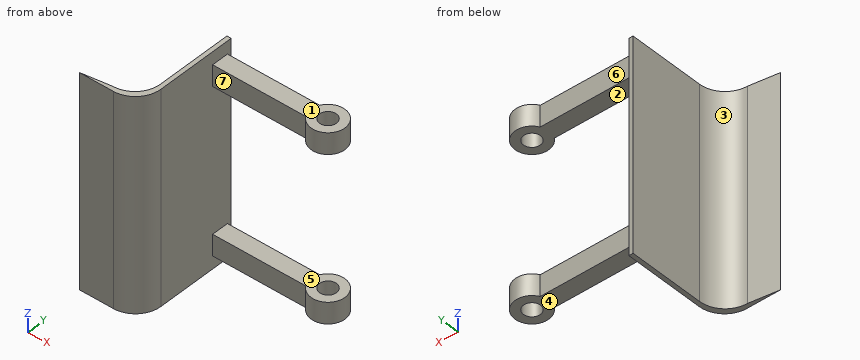
from build123d import *

# Parameters (mm, degrees)
BOSS_EXTRU_1_DEPTH      = 250
ESQUISSE3_W             = 25
ESQUISSE3_H             = 20
BOSS_EXTRU_2_DEPTH      = 125
ESQUISSE4_R             = 20
BOSS_EXTRU_3_DEPTH      = 25
ESQUISSE5_R             = 20
BOSS_EXTRU_4_DEPTH      = 25
ESQUISSE6_R             = 10
ENL_V_MAT_EXTRU_1_DEPTH = 236


with BuildPart() as part:
    # Esquisse1 → Boss.-Extru.1 (new body)
    with BuildSketch(Plane.XY):
        with BuildLine():
            Line((-30, 0), (-69.925793841, 0))
            Line((-69.925793841, 0), (-35, 5))
            ThreePointArc((-35, 5), (-13.786796564, 13.786796564), (-5, 35))
            Line((-5, 35), (-5, 125))
            Line((-5, 125), (0, 125))
            Line((0, 125), (0, 30))
            ThreePointArc((0, 30), (-8.786796564, 8.786796564), (-30, 0))
        make_face()
    extrude(amount=BOSS_EXTRU_1_DEPTH)

    # Esquisse3 → Boss.-Extru.2 (add)
    with BuildSketch(Plane(origin=(0, 0, 0), x_dir=(0, 0, -1), z_dir=(1, 0, 0))):
        with Locations((-222.5, 110)):
            Rectangle(ESQUISSE3_W, ESQUISSE3_H)
        with Locations((-27.5, 110)):
            Rectangle(ESQUISSE3_W, ESQUISSE3_H)
    extrude(amount=BOSS_EXTRU_2_DEPTH)

    # Esquisse4 → Boss.-Extru.3 (add)
    with BuildSketch(Plane.XY.offset(235)):
        with Locations((127, 110.778032317)):
            Circle(ESQUISSE4_R)
    extrude(amount=-BOSS_EXTRU_3_DEPTH)

    # Esquisse5 → Boss.-Extru.4 (add)
    with BuildSketch(Plane.XY.offset(40)):
        with Locations((127, 110.778032317)):
            Circle(ESQUISSE5_R)
    extrude(amount=-BOSS_EXTRU_4_DEPTH)

    # Esquisse6 → Enlèv. mat.-Extru.1 (cut, through all)
    with BuildSketch(Plane.XY.offset(235)):
        with Locations((127, 110.778032317)):
            Circle(ESQUISSE6_R)
    extrude(amount=-ENL_V_MAT_EXTRU_1_DEPTH, mode=Mode.SUBTRACT)


solid = part.part
Source: CAD feature listing. Evaluate the final solid. Frame: model axes, mm. Face numbers are marked on the shaded views. A direction names the side the tool comes from. Round coordinates to 2 decimals unless told otherwise and drop trailing zeros. Loops run counter-clockwise (first coordinate to the right, second up) from the corner with the lowest first, then second, coordinate; pieces in that order, holes last. Notation, with made-up numbers: (72.25, -7) -> (131.25, -7) arc R10 cw to (131.25, 8) -> close; hole circle Ø1 at (35, 63.5). An arc over 180 degrees is marked (long way). Answer as a JSON object with one key per item and string values. Group by question number.
Q1. Mould query, pull axis Z, two halves, no side actions, for the marked faces 1, 2, 3 and 4. Classes: pulls with the +Z half, pulls with the -Z half, needs draft (parallel to the pull), parting line crosses it, or undercut.
Q2. Contact query for flat-ended pins moving along their axis: P1, Ø6, axis at y = 87, z = 38, coming from the +X side; P2, Ø7.5, axis at x = 72.5, z = 29.5, coming from the -Y side; P3, Ø4, axis at x = 106, z = 224, coming from the +Y side. Output: stop coordinate, or through.
Q3. Section query B-B (x = 38.5). Output: boundary loops of the cut face in (y, z), plus the area to 3 significant figures.
Q4. Ray query, line 1 (Y direction, x = 127, z = 224.5); line 2 (Z direction, x = 118, y = 99.5); line 3 (X direction, y = 45.5, z = 50.5). Return the intervals inside material, ascending. Write a range as from..to.
Q5. Section query D-D (y = 53). Output: boundary loops of the cut face in (x, z), plus the area to 3 significant figures.
Q6. Access query for the marked faces 5, 6 and 7. Directions: +Z, -Z, +X, -X, +Y, -Y. A direction counts if a zero-diameter tool reaches every point of the face in a straight line with its end or side. Return the directions, or none.
Q7. Section query A-A (x = 127). Output: boundary loops of the cut face in (y, z), plus the area to 3 significant figures.
Q8. Section query C-C (z = 170.5). Output: boundary loops of the cut face in (x, y).
Completed:
{
 "1": {"face 1": "pulls with the +Z half", "face 2": "undercut", "face 3": "needs draft", "face 4": "pulls with the -Z half"},
 "2": {"P1": "x = 0", "P2": "y = 100", "P3": "y = 120"},
 "3": {"outline": "(100, 15) -> (120, 15) -> (120, 40) -> (100, 40) -> close; (100, 210) -> (120, 210) -> (120, 235) -> (100, 235) -> close", "area": "1,000 mm²"},
 "4": {"line 1": "90.78..100.78, 120.78..130.78", "line 2": "15..40, 210..235", "line 3": "-5..0"},
 "5": {"outline": "(-5, 0) -> (0, 0) -> (0, 250) -> (-5, 250) -> close", "area": "1,250 mm²"},
 "6": {"face 5": "+X, +Y, -Y", "face 6": "+Z, -Z, +Y", "face 7": "+Z, -Z, -Y"},
 "7": {"outline": "(90.78, 15) -> (100.78, 15) -> (100.78, 40) -> (90.78, 40) -> close; (90.78, 210) -> (100.78, 210) -> (100.78, 235) -> (90.78, 235) -> close; (120.78, 15) -> (130.78, 15) -> (130.78, 40) -> (120.78, 40) -> close; (120.78, 210) -> (130.78, 210) -> (130.78, 235) -> (120.78, 235) -> close", "area": "1,000 mm²"},
 "8": {"outline": "(-69.93, 0) -> (-30, 0) arc R30 ccw to (0, 30) -> (0, 125) -> (-5, 125) -> (-5, 35) arc R30 cw to (-35, 5) -> close"}
}
